Check sheet for the modelled part. Datum: model origin and axes. Units: mm. Coordinates: 2 decimals unless noted, no trailing zeros. Order: outer loops, then holes, each group sorted by start corner. A loop starts at its lowest first (then second) coordinate and runs counter-clockwise, first axis right, second up.
1. Cross-section at C-C (y = 4.95). Enter the section's corners in (x, z) (3 decimals), then the cut area to 3 significant figures.
2. Cross-section at A-A (x = 0). Enter the section's corners in (y, z) (3 decimals), then the cut area to 3 significant figures.
3. Thickness scan on line 1 (Z direction, x = 0, y = 1.55) (3 decimals); line 2 (X direction, y = 5.15, z = 3); line 3 (Z direction, x = -3, y = 1.45) (3 decimals). Record the ranges inside material, lowest first.
4. Cross-section at B-B (y = 1.6). Enter the section's corners in (x, z) (3 decimals), then the cut area to 3 significant figures.
5. Gauge pin test, flat ends, axial feed: pin 1 Ø1.5 at (y, z) = (2, 2) entering from +X; pin 2 Ø1.5 at (x, z) = (2.5, 0) entering from -Y; pin 3 Ø1 at (y, z) = (3.5, -3.5) entering from -X; pin 4 Ø1.5 at (y, z) = (2, 1) entering from +X. Record the tip position at first contact, or that the pin passes through.
6. Draft check along Z on faces 1 (the flat face through (0, 3, 6.225)), 2 (the flat face through (0, 3, -6.225)), 3 (the cylindrical face through (-0.818, 2.958, 3.685)). Enter one of: released by +Z, released by -Z, zero draft, split by the parting line, or undercut.
```python
from build123d import *

# Parameters (mm, degrees)
SKETCH1_R           = 3.775
BOSS_EXTRUDE1_DEPTH = 6


with BuildPart() as part:
    # Sketch1 → Boss-Extrude1 (new body)
    with BuildSketch(Plane(origin=(0, 0, 0), x_dir=(1, 0, 0), z_dir=(0, 1, 0))):
        Polygon((-7.188010851, 0), (-3.594005426, -6.225), (3.594005426, -6.225), (7.188010851, 0), (3.594005426, 6.225), (-3.594005426, 6.225), align=None)
        Circle(SKETCH1_R, mode=Mode.SUBTRACT)
    extrude(amount=BOSS_EXTRUDE1_DEPTH)

    # Sketch5 → Cut-Revolve1 (revolve, cut)
    with BuildSketch(Plane.XY):
        Polygon((-5.938010851, 6), (-7.188010851, 6), (-7.188010851, 4.75), align=None)
        Polygon((-5.938010851, 0), (-7.188010851, 0), (-7.188010851, 1.25), align=None)
    revolve(axis=Axis((0, 0, 0), (0, 1, 0)), mode=Mode.SUBTRACT)


solid = part.part
```
Data:
1. outline: (-6.979, -0.363) - (-3.803, -5.862) arc R6.988 ccw to (-3.175, -6.225) - (3.175, -6.225) arc R6.988 ccw to (3.803, -5.862) - (6.979, -0.363) arc R6.988 ccw to (6.979, 0.363) - (3.803, 5.862) arc R6.988 ccw to (3.175, 6.225) - (-3.175, 6.225) arc R6.988 ccw to (-3.803, 5.862) - (-6.979, 0.363) arc R6.988 ccw to start; hole circle Ø7.55 at (0, 0)
1. area: 89.0 mm2
2. outline: (0, -5.938) - (0.287, -6.225) - (5.713, -6.225) - (6, -5.938) - (6, -3.775) - (0, -3.775) - close; (0, 3.775) - (6, 3.775) - (6, 5.938) - (5.713, 6.225) - (0.287, 6.225) - (0, 5.938) - close
2. area: 29.2 mm2
3. line 1: z = -6.225 to -3.775, 3.775 to 6.225
3. line 2: x = -5.46 to -2.29, 2.29 to 5.46
3. line 3: z = -6.225 to -2.291, 2.291 to 6.225
4. outline: (-7.188, 0) - (-3.594, -6.225) - (3.594, -6.225) - (7.188, 0) - (3.594, 6.225) - (-3.594, 6.225) - close; hole circle Ø7.55 at (0, 0)
4. area: 89.5 mm2
5. pin 1: stops at x = 6.47
5. pin 2: passes through
5. pin 3: stops at x = -5.46
5. pin 4: stops at x = 7.04
6. face 1: released by +Z
6. face 2: released by -Z
6. face 3: undercut
